from build123d import *

# Parameters (mm, degrees)
BOSS_EXTRUDE1_DEPTH                          = 2
FILLET1_R                                    = 3
CUT_EXTRUDE1_REACH                           = 58.767
SKETCH2_R                                    = 1.25
CIRPATTERN1_COUNT                            = 8
CUT_EXTRUDE2_REACH                           = 58.767
SKETCH3_R                                    = 1.35
SKETCH3_R_2                                  = 1.25
SKETCH3_R_3                                  = 2.5
MIRROR1_AT_THE_SECOND_PLANE_COPY_1_REACH     = 58.767
MIRROR1_AT_THE_SECOND_PLANE_COPY_1_SKETC_R   = 1.35
MIRROR1_AT_THE_SECOND_PLANE_COPY_1_SKETC_R_2 = 1.25
MIRROR1_AT_THE_SECOND_PLANE_COPY_1_SKETC_R_3 = 2.5


with BuildPart() as part:
    # Sketch1 → Boss-Extrude1 (new body)
    with BuildSketch(Plane(origin=(0, 0, 0), x_dir=(1, 0, 0), z_dir=(0, 1, 0))):
        Polygon((9, 26), (-9, 26), (-9, 46.5), (-32.5, 46.5), (-32.5, -46.5), (-9, -46.5), (-9, -26), (9, -26), (9, -46.5), (32.5, -46.5), (32.5, 46.5), (9, 46.5), align=None)
    extrude(amount=BOSS_EXTRUDE1_DEPTH)

    # Fillet1
    fillet1_edges = [part.edges().sort_by_distance(p)[0] for p in [
        (-9, 1, -26),
        (9, 1, -26),
        (9, 1, -46.5),
        (32.5, 1, -46.5),
        (32.5, 1, 46.5),
        (9, 1, 46.5),
        (9, 1, 26),
        (-9, 1, 26),
        (-9, 1, 46.5),
        (-32.5, 1, 46.5),
        (-32.5, 1, -46.5),
        (-9, 1, -46.5),
    ]]
    fillet(fillet1_edges, radius=FILLET1_R)

    # Sketch2 → Cut-Extrude1 (cut, up to next)
    with BuildSketch(Plane(origin=(0, 2, 0), x_dir=(1, 0, 0), z_dir=(0, 1, 0)), mode=Mode.PRIVATE) as cut_extrude1_sk1:
        with Locations(Location((0, 0, 0), (0, 0, 270))):
            Circle(SKETCH2_R)
    cut_extrude1_tool1 = extrude(cut_extrude1_sk1.sketch, amount=-CUT_EXTRUDE1_REACH, mode=Mode.PRIVATE) & part.part
    # Sketch2 → Cut-Extrude1 (cut, up to next)
    with BuildSketch(Plane(origin=(0, 2, 0), x_dir=(1, 0, 0), z_dir=(0, 1, 0)), mode=Mode.PRIVATE) as cut_extrude1_sk2:
        with BuildLine():
            Line((0.5, 21.125), (-0.5, 21.125))
            ThreePointArc((-0.5, 21.125), (-1.207106781, 20.832106781), (-1.5, 20.125))
            Line((-1.5, 20.125), (-1.5, 7.125))
            ThreePointArc((-1.5, 7.125), (-1.207106781, 6.417893219), (-0.5, 6.125))
            Line((-0.5, 6.125), (0.5, 6.125))
            ThreePointArc((0.5, 6.125), (1.207106781, 6.417893219), (1.5, 7.125))
            Line((1.5, 7.125), (1.5, 20.125))
            ThreePointArc((1.5, 20.125), (1.207106781, 20.832106781), (0.5, 21.125))
        make_face()
    cut_extrude1_tool2 = extrude(cut_extrude1_sk2.sketch, amount=-CUT_EXTRUDE1_REACH, mode=Mode.PRIVATE) & part.part
    cut_extrude1_1 = cut_extrude1_tool1.solids().sort_by_distance((0, 2, 0))[0]
    add(cut_extrude1_1, mode=Mode.SUBTRACT)
    cut_extrude1_2 = cut_extrude1_tool2.solids().sort_by_distance((0, 2, -13.625))[0]
    add(cut_extrude1_2, mode=Mode.SUBTRACT)
    cut_extrude1 = cut_extrude1_1 + cut_extrude1_2  # Cut-Extrude1 as one shape, for the pattern or mirror that repeats it

    # CirPattern1: Cut-Extrude1 ×8 about axis
    cirpattern1_axis = Axis((0, 0, 0), (0, 1, 0))
    for i in range(1, CIRPATTERN1_COUNT):
        add(cut_extrude1.rotate(cirpattern1_axis, i * 360 / CIRPATTERN1_COUNT), mode=Mode.SUBTRACT)

    # Sketch3 → Cut-Extrude2 (cut, up to next)
    with BuildSketch(Plane(origin=(0, 2, 0), x_dir=(1, 0, 0), z_dir=(0, 1, 0)), mode=Mode.PRIVATE) as cut_extrude2_sk1:
        with Locations(Location((-29.5, 43.5, 0), (0, 0, 270))):
            Circle(SKETCH3_R)
    cut_extrude2_tool1 = extrude(cut_extrude2_sk1.sketch, amount=-CUT_EXTRUDE2_REACH, mode=Mode.PRIVATE) & part.part
    # Sketch3 → Cut-Extrude2 (cut, up to next)
    with BuildSketch(Plane(origin=(0, 2, 0), x_dir=(1, 0, 0), z_dir=(0, 1, 0)), mode=Mode.PRIVATE) as cut_extrude2_sk2:
        with Locations(Location((-24.5, 40.5, 0), (0, 0, 270))):
            Circle(SKETCH3_R)
    cut_extrude2_tool2 = extrude(cut_extrude2_sk2.sketch, amount=-CUT_EXTRUDE2_REACH, mode=Mode.PRIVATE) & part.part
    # Sketch3 → Cut-Extrude2 (cut, up to next)
    with BuildSketch(Plane(origin=(0, 2, 0), x_dir=(1, 0, 0), z_dir=(0, 1, 0)), mode=Mode.PRIVATE) as cut_extrude2_sk3:
        with Locations(Location((-24.5, 18, 0), (0, 0, 270))):
            Circle(SKETCH3_R_2)
    cut_extrude2_tool3 = extrude(cut_extrude2_sk3.sketch, amount=-CUT_EXTRUDE2_REACH, mode=Mode.PRIVATE) & part.part
    # Sketch3 → Cut-Extrude2 (cut, up to next)
    with BuildSketch(Plane(origin=(0, 2, 0), x_dir=(1, 0, 0), z_dir=(0, 1, 0)), mode=Mode.PRIVATE) as cut_extrude2_sk4:
        with Locations(Location((-18.5, 37, 0), (0, 0, 270))):
            Circle(SKETCH3_R)
    cut_extrude2_tool4 = extrude(cut_extrude2_sk4.sketch, amount=-CUT_EXTRUDE2_REACH, mode=Mode.PRIVATE) & part.part
    # Sketch3 → Cut-Extrude2 (cut, up to next)
    with BuildSketch(Plane(origin=(0, 2, 0), x_dir=(1, 0, 0), z_dir=(0, 1, 0)), mode=Mode.PRIVATE) as cut_extrude2_sk5:
        with Locations(Location((-18.5, 23, 0), (0, 0, 270))):
            Circle(SKETCH3_R)
    cut_extrude2_tool5 = extrude(cut_extrude2_sk5.sketch, amount=-CUT_EXTRUDE2_REACH, mode=Mode.PRIVATE) & part.part
    # Sketch3 → Cut-Extrude2 (cut, up to next)
    with BuildSketch(Plane(origin=(0, 2, 0), x_dir=(1, 0, 0), z_dir=(0, 1, 0)), mode=Mode.PRIVATE) as cut_extrude2_sk6:
        with Locations(Location((-18.5, 30, 0), (0, 0, 270))):
            Circle(SKETCH3_R_3)
    cut_extrude2_tool6 = extrude(cut_extrude2_sk6.sketch, amount=-CUT_EXTRUDE2_REACH, mode=Mode.PRIVATE) & part.part
    cut_extrude2_1 = cut_extrude2_tool1.solids().sort_by_distance((-29.5, 2, -43.5))[0]
    add(cut_extrude2_1, mode=Mode.SUBTRACT)
    cut_extrude2_2 = cut_extrude2_tool2.solids().sort_by_distance((-24.5, 2, -40.5))[0]
    add(cut_extrude2_2, mode=Mode.SUBTRACT)
    cut_extrude2_3 = cut_extrude2_tool3.solids().sort_by_distance((-24.5, 2, -18))[0]
    add(cut_extrude2_3, mode=Mode.SUBTRACT)
    cut_extrude2_4 = cut_extrude2_tool4.solids().sort_by_distance((-18.5, 2, -37))[0]
    add(cut_extrude2_4, mode=Mode.SUBTRACT)
    cut_extrude2_5 = cut_extrude2_tool5.solids().sort_by_distance((-18.5, 2, -23))[0]
    add(cut_extrude2_5, mode=Mode.SUBTRACT)
    cut_extrude2_6 = cut_extrude2_tool6.solids().sort_by_distance((-18.5, 2, -30))[0]
    add(cut_extrude2_6, mode=Mode.SUBTRACT)
    cut_extrude2 = cut_extrude2_1 + cut_extrude2_2 + cut_extrude2_3 + cut_extrude2_4 + cut_extrude2_5 + cut_extrude2_6  # Cut-Extrude2 as one shape, for the pattern or mirror that repeats it

    # Mirror1: Cut-Extrude2 across plane
    add(cut_extrude2.mirror(Plane(origin=(0, 0, 0), x_dir=(0, 0, 1), z_dir=(1, 0, 0))), mode=Mode.SUBTRACT)

    # Mirror1 at the second plane: Cut-Extrude2 across plane
    add(cut_extrude2.mirror(Plane.XY), mode=Mode.SUBTRACT)

    # Mirror1 at the second plane copy 1 sketc → Mirror1 at the second plane copy 1 (cut, up to next)
    with BuildSketch(Plane(origin=(0, 2, 0), x_dir=(-1, 0, 0), z_dir=(0, 1, 0)), mode=Mode.PRIVATE) as mirror1_at_the_second_plane_copy_1_sk1:
        with Locations(Location((-29.5, 43.5, 0), (0, 0, 270))):
            Circle(MIRROR1_AT_THE_SECOND_PLANE_COPY_1_SKETC_R)
    mirror1_at_the_second_plane_copy_1_tool1 = extrude(mirror1_at_the_second_plane_copy_1_sk1.sketch, amount=-MIRROR1_AT_THE_SECOND_PLANE_COPY_1_REACH, mode=Mode.PRIVATE) & part.part
    # Mirror1 at the second plane copy 1 sketc → Mirror1 at the second plane copy 1 (cut, up to next)
    with BuildSketch(Plane(origin=(0, 2, 0), x_dir=(-1, 0, 0), z_dir=(0, 1, 0)), mode=Mode.PRIVATE) as mirror1_at_the_second_plane_copy_1_sk2:
        with Locations(Location((-24.5, 40.5, 0), (0, 0, 270))):
            Circle(MIRROR1_AT_THE_SECOND_PLANE_COPY_1_SKETC_R)
    mirror1_at_the_second_plane_copy_1_tool2 = extrude(mirror1_at_the_second_plane_copy_1_sk2.sketch, amount=-MIRROR1_AT_THE_SECOND_PLANE_COPY_1_REACH, mode=Mode.PRIVATE) & part.part
    # Mirror1 at the second plane copy 1 sketc → Mirror1 at the second plane copy 1 (cut, up to next)
    with BuildSketch(Plane(origin=(0, 2, 0), x_dir=(-1, 0, 0), z_dir=(0, 1, 0)), mode=Mode.PRIVATE) as mirror1_at_the_second_plane_copy_1_sk3:
        with Locations(Location((-24.5, 18, 0), (0, 0, 270))):
            Circle(MIRROR1_AT_THE_SECOND_PLANE_COPY_1_SKETC_R_2)
    mirror1_at_the_second_plane_copy_1_tool3 = extrude(mirror1_at_the_second_plane_copy_1_sk3.sketch, amount=-MIRROR1_AT_THE_SECOND_PLANE_COPY_1_REACH, mode=Mode.PRIVATE) & part.part
    # Mirror1 at the second plane copy 1 sketc → Mirror1 at the second plane copy 1 (cut, up to next)
    with BuildSketch(Plane(origin=(0, 2, 0), x_dir=(-1, 0, 0), z_dir=(0, 1, 0)), mode=Mode.PRIVATE) as mirror1_at_the_second_plane_copy_1_sk4:
        with Locations(Location((-18.5, 37, 0), (0, 0, 270))):
            Circle(MIRROR1_AT_THE_SECOND_PLANE_COPY_1_SKETC_R)
    mirror1_at_the_second_plane_copy_1_tool4 = extrude(mirror1_at_the_second_plane_copy_1_sk4.sketch, amount=-MIRROR1_AT_THE_SECOND_PLANE_COPY_1_REACH, mode=Mode.PRIVATE) & part.part
    # Mirror1 at the second plane copy 1 sketc → Mirror1 at the second plane copy 1 (cut, up to next)
    with BuildSketch(Plane(origin=(0, 2, 0), x_dir=(-1, 0, 0), z_dir=(0, 1, 0)), mode=Mode.PRIVATE) as mirror1_at_the_second_plane_copy_1_sk5:
        with Locations(Location((-18.5, 23, 0), (0, 0, 270))):
            Circle(MIRROR1_AT_THE_SECOND_PLANE_COPY_1_SKETC_R)
    mirror1_at_the_second_plane_copy_1_tool5 = extrude(mirror1_at_the_second_plane_copy_1_sk5.sketch, amount=-MIRROR1_AT_THE_SECOND_PLANE_COPY_1_REACH, mode=Mode.PRIVATE) & part.part
    # Mirror1 at the second plane copy 1 sketc → Mirror1 at the second plane copy 1 (cut, up to next)
    with BuildSketch(Plane(origin=(0, 2, 0), x_dir=(-1, 0, 0), z_dir=(0, 1, 0)), mode=Mode.PRIVATE) as mirror1_at_the_second_plane_copy_1_sk6:
        with Locations(Location((-18.5, 30, 0), (0, 0, 270))):
            Circle(MIRROR1_AT_THE_SECOND_PLANE_COPY_1_SKETC_R_3)
    mirror1_at_the_second_plane_copy_1_tool6 = extrude(mirror1_at_the_second_plane_copy_1_sk6.sketch, amount=-MIRROR1_AT_THE_SECOND_PLANE_COPY_1_REACH, mode=Mode.PRIVATE) & part.part
    add(mirror1_at_the_second_plane_copy_1_tool1.solids().sort_by_distance((29.5, 2, 43.5))[0], mode=Mode.SUBTRACT)
    add(mirror1_at_the_second_plane_copy_1_tool2.solids().sort_by_distance((24.5, 2, 40.5))[0], mode=Mode.SUBTRACT)
    add(mirror1_at_the_second_plane_copy_1_tool3.solids().sort_by_distance((24.5, 2, 18))[0], mode=Mode.SUBTRACT)
    add(mirror1_at_the_second_plane_copy_1_tool4.solids().sort_by_distance((18.5, 2, 37))[0], mode=Mode.SUBTRACT)
    add(mirror1_at_the_second_plane_copy_1_tool5.solids().sort_by_distance((18.5, 2, 23))[0], mode=Mode.SUBTRACT)
    add(mirror1_at_the_second_plane_copy_1_tool6.solids().sort_by_distance((18.5, 2, 30))[0], mode=Mode.SUBTRACT)


solid = part.part
Part model, mm, in its own coordinate system. A direction names the side the tool comes from. Coordinates: 2 decimals unless noted, no trailing zeros. Loops run counter-clockwise (first coordinate to the right, second up) from the corner with the lowest first, then second, coordinate; pieces in that order, holes last. Notation, with made-up numbers: (29, 33) -> (69, 33) arc R23 cw to (69, 55) -> close; hole circle Ø3 at (50, 53). An arc over 180 degrees is marked (long way). Use a Markdown table: item, result. Add a question column.
Item 1: Band-saw the part on B-B on z = -34. Write the cut outline in (x, y).
Item 2: Which spindle directions (+Z, -Z, +X, -X, +Y, -Y) get a long thin tool onto all of the face, cutting with end or side? Do faces 1 (the flat face through (14, 1, -1.5)), 2 (the flat face through (7, 2, -11)), 3 (the flat face through (-9, 1, -36)). Say none if no direction does.
Item 3: Band-saw the part on A-A on x = -18.5. Give the number of separate pieces and of enclosed holes in the cut face, plus the area to 3 significant figures.
Item 4: Pull direction Z, two halves, no side cores. Call faces 4 (the flat face through (-1.5, 1, 14)), 5 (the cylindrical face through (-8.14, 1.01, 26.9)), 6 (the flat face through (9, 1, 36)): +Z half, -Z half, draft (parallel to the pull), parting line (faces both ways), or undercut.
Item 5: Band-saw the part on D-D on z = 37. Write the cut outline in (x, y), plus the area to 3 significant figures.
Item 6: Band-saw the part on C-C on z = -23. Write the cut outline in (x, y).
Item 7: Probe probe 1 along X at (y, z) = (0.8, 40.5); probe 2 along X at (y, z) = (1.4, 30); probe 3 along X at (y, z) = (1.4, -4). List the from-to ranges inside material, lowest first.
Geometry says:
| question | item | result |
|---|---|---|
| 1 | outline | (-32.5, 0) -> (-9, 0) -> (-9, 2) -> (-32.5, 2) -> close; (9, 0) -> (32.5, 0) -> (32.5, 2) -> (9, 2) -> close |
| 2 | face 1 | +Y, -Y |
| 2 | face 2 | +Z, -Z, +X, -X, +Y |
| 2 | face 3 | -Z, +Y, -Y |
| 3 | separate pieces | 8 |
| 3 | enclosed holes | 0 |
| 3 | area | 138 mm² |
| 4 | face 4 | undercut |
| 4 | face 5 | +Z half |
| 4 | face 6 | draft |
| 5 | outline | (-32.5, 0) -> (-19.85, 0) -> (-19.85, 2) -> (-32.5, 2) -> close; (-17.15, 0) -> (-9, 0) -> (-9, 2) -> (-17.15, 2) -> close; (9, 0) -> (17.15, 0) -> (17.15, 2) -> (9, 2) -> close; (19.85, 0) -> (32.5, 0) -> (32.5, 2) -> (19.85, 2) -> close |
| 5 | area | 83.2 mm² |
| 6 | outline | (-32.5, 0) -> (-19.85, 0) -> (-19.85, 2) -> (-32.5, 2) -> close; (-17.15, 0) -> (17.15, 0) -> (17.15, 2) -> (-17.15, 2) -> close; (19.85, 0) -> (32.5, 0) -> (32.5, 2) -> (19.85, 2) -> close |
| 7 | probe 1 | -32.5 to -25.85, -23.15 to -9, 9 to 23.15, 25.85 to 32.5 |
| 7 | probe 2 | -32.5 to -21, -16 to -9, 9 to 16, 21 to 32.5 |
| 7 | probe 3 | -32.5 to -6.12, -4.66 to 4.66, 6.12 to 32.5 |
